Autodesk Inventor part; units mm, degrees
ref_plane "YZ Plane" through (0, 0, 0) normal (1, 0, 0) x (0, 1, 0)
ref_plane "XZ Plane" through (0, 0, 0) normal (0, 1, 0) x (-1, 0, 0)
ref_plane "XY Plane" through (0, 0, 0) normal (0, 0, 1) x (1, 0, 0)
sketch "Sketch1" plane through (0, 0, 0) normal (0, 1, 0) x (-1, 0, 0)
  line L0 (0, 0) -> (878.84, 0)
  line L1 (878.84, 0) -> (878.84, -66.04)
  line L2 (878.84, -66.04) -> (0, -66.04)
  line L3 (0, -66.04) -> (0, 0)
  line L4 (0, 0) -> (0, -20.32)
  line L5 (0, 0) -> (20.32, 0) construction
  line L6 (0, -20.32) -> (878.84, -20.32)
  line L7 (0, -10.16) -> (20.32, -10.16)
  line L8 (0, -10.16) -> (20.32, -10.16) construction
  circle A0 centre (20.32, -10.16) radius 2.54
  line L9 (20.32, -10.16) -> (172.72, -10.16)
  line L10 (20.32, -10.16) -> (172.72, -10.16) construction
  circle A1 centre (172.72, -10.16) radius 2.54
  line L11 (172.72, -10.16) -> (325.12, -10.16)
  circle A2 centre (325.12, -10.16) radius 2.54
  line L12 (325.12, -10.16) -> (477.52, -10.16)
  circle A3 centre (477.52, -10.16) radius 2.54
  line L13 (477.52, -10.16) -> (629.92, -10.16)
  circle A4 centre (629.92, -10.16) radius 2.54
  line L14 (629.92, -10.16) -> (782.32, -10.16)
  circle A5 centre (782.32, -10.16) radius 2.54
  line L15 (878.84, 0) -> (878.84, -10.16)
  line L16 (878.84, 0) -> (889, 0) construction
  line L17 (878.84, -10.16) -> (868.68, -10.16)
  circle A6 centre (868.68, -10.16) radius 2.54
  line L18 (0, 0) -> (0, -27.94)
  line L19 (0, 0) -> (27.94, 0) construction
  line L20 (0, -27.94) -> (27.94, -27.94)
  circle A7 centre (27.94, -27.94) radius 2.54
  line L21 (27.94, -27.94) -> (104.14, -27.94)
  line L22 (27.94, -27.94) -> (104.14, -27.94) construction
  circle A8 centre (104.14, -27.94) radius 2.54
  line L23 (104.14, -27.94) -> (129.54, -27.94)
  line L24 (142.24, -40.64) -> (142.24, -66.04)
  line L25 (142.24, -66.04) -> (116.84, -66.04)
  line L26 (116.84, -66.04) -> (116.84, -40.64)
  line L27 (116.84, -27.94) -> (116.84, -40.64)
  line L28 (116.84, -27.94) -> (129.54, -27.94) construction
  line L29 (116.84, -40.64) -> (129.54, -40.64)
  arc A9 (142.24, -40.64) -> (116.84, -40.64) centre (129.54, -40.64) ccw
  line L30 (142.24, -40.64) -> (154.94, -40.64) construction
  line L31 (142.24, -66.04) -> (154.94, -66.04)
  line L32 (142.24, -66.04) -> (154.94, -66.04) construction
  line L33 (154.94, -66.04) -> (154.94, -34.29)
  circle A10 centre (154.94, -34.29) radius 2.54
  line L34 (154.94, -34.29) -> (231.14, -34.29)
  line L35 (154.94, -34.29) -> (231.14, -34.29) construction
  circle A11 centre (231.14, -34.29) radius 2.54
  line L36 (154.94, -34.29) -> (104.14, -34.29)
  line L37 (154.94, -34.29) -> (205.74, -34.29) construction
  line L38 (269.24, -40.64) -> (269.24, -66.04)
  line L39 (243.84, -66.04) -> (243.84, -40.64)
  arc A12 (269.24, -40.64) -> (243.84, -40.64) centre (256.54, -40.64) ccw
  circle A13 centre (281.94, -34.29) radius 2.54
  line L40 (281.94, -34.29) -> (358.14, -34.29)
  circle A14 centre (358.14, -34.29) radius 2.54
  line L41 (281.94, -34.29) -> (231.14, -34.29)
  line L42 (396.24, -40.64) -> (396.24, -66.04)
  line L43 (370.84, -66.04) -> (370.84, -40.64)
  arc A15 (396.24, -40.64) -> (370.84, -40.64) centre (383.54, -40.64) ccw
  circle A16 centre (408.94, -34.29) radius 2.54
  line L44 (408.94, -34.29) -> (485.14, -34.29)
  circle A17 centre (485.14, -34.29) radius 2.54
  line L45 (408.94, -34.29) -> (358.14, -34.29)
  line L46 (523.24, -40.64) -> (523.24, -66.04)
  line L47 (497.84, -66.04) -> (497.84, -40.64)
  arc A18 (523.24, -40.64) -> (497.84, -40.64) centre (510.54, -40.64) ccw
  circle A19 centre (535.94, -34.29) radius 2.54
  line L48 (535.94, -34.29) -> (612.14, -34.29)
  circle A20 centre (612.14, -34.29) radius 2.54
  line L49 (535.94, -34.29) -> (485.14, -34.29)
  line L50 (650.24, -40.64) -> (650.24, -66.04)
  line L51 (624.84, -66.04) -> (624.84, -40.64)
  arc A21 (650.24, -40.64) -> (624.84, -40.64) centre (637.54, -40.64) ccw
  circle A22 centre (662.94, -34.29) radius 2.54
  line L52 (662.94, -34.29) -> (739.14, -34.29)
  circle A23 centre (739.14, -34.29) radius 2.54
  line L53 (662.94, -34.29) -> (612.14, -34.29)
  line L54 (777.24, -40.64) -> (777.24, -66.04)
  line L55 (751.84, -66.04) -> (751.84, -40.64)
  arc A24 (777.24, -40.64) -> (751.84, -40.64) centre (764.54, -40.64) ccw
  circle A25 centre (789.94, -34.29) radius 2.54
  line L56 (789.94, -34.29) -> (866.14, -34.29)
  circle A26 centre (866.14, -34.29) radius 2.54
  line L57 (789.94, -34.29) -> (739.14, -34.29)
  line L58 (0, -132.08) -> (878.84, -132.08)
  line L59 (878.84, -132.08) -> (878.84, -66.04)
  line L60 (0, -66.04) -> (0, -132.08)
  line L61 (0, -132.08) -> (0, -111.76)
  line L62 (0, -132.08) -> (20.32, -132.08) construction
  line L63 (0, -111.76) -> (878.84, -111.76)
  line L64 (0, -121.92) -> (20.32, -121.92)
  line L65 (0, -121.92) -> (20.32, -121.92) construction
  circle A27 centre (20.32, -121.92) radius 2.54
  line L66 (20.32, -121.92) -> (172.72, -121.92)
  line L67 (20.32, -121.92) -> (172.72, -121.92) construction
  circle A28 centre (172.72, -121.92) radius 2.54
  circle A29 centre (325.12, -121.92) radius 2.54
  line L68 (172.72, -121.92) -> (325.12, -121.92)
  circle A30 centre (477.52, -121.92) radius 2.54
  line L69 (325.12, -121.92) -> (477.52, -121.92)
  circle A31 centre (629.92, -121.92) radius 2.54
  line L70 (477.52, -121.92) -> (629.92, -121.92)
  circle A32 centre (782.32, -121.92) radius 2.54
  line L71 (629.92, -121.92) -> (782.32, -121.92)
  line L72 (878.84, -132.08) -> (878.84, -121.92)
  line L73 (878.84, -132.08) -> (889, -132.08) construction
  line L74 (878.84, -121.92) -> (868.68, -121.92)
  circle A33 centre (868.68, -121.92) radius 2.54
  line L75 (0, -132.08) -> (0, -104.14)
  line L76 (0, -132.08) -> (27.94, -132.08) construction
  line L77 (0, -104.14) -> (27.94, -104.14)
  circle A34 centre (27.94, -104.14) radius 2.54
  line L78 (27.94, -104.14) -> (104.14, -104.14)
  line L79 (27.94, -104.14) -> (104.14, -104.14) construction
  circle A35 centre (104.14, -104.14) radius 2.54
  line L80 (104.14, -104.14) -> (129.54, -104.14)
  line L81 (142.24, -91.44) -> (142.24, -66.04)
  line L82 (116.84, -66.04) -> (116.84, -91.44)
  line L83 (116.84, -104.14) -> (116.84, -91.44)
  line L84 (116.84, -104.14) -> (129.54, -104.14) construction
  line L85 (116.84, -91.44) -> (129.54, -91.44)
  arc A36 (116.84, -91.44) -> (142.24, -91.44) centre (129.54, -91.44) ccw
  line L86 (142.24, -91.44) -> (154.94, -91.44) construction
  line L87 (154.94, -66.04) -> (154.94, -97.79)
  circle A37 centre (154.94, -97.79) radius 2.54
  line L88 (154.94, -97.79) -> (231.14, -97.79)
  line L89 (154.94, -97.79) -> (231.14, -97.79) construction
  circle A38 centre (231.14, -97.79) radius 2.54
  line L90 (154.94, -97.79) -> (104.14, -97.79)
  line L91 (154.94, -97.79) -> (205.74, -97.79) construction
  line L92 (281.94, -97.79) -> (231.14, -97.79)
  line L93 (281.94, -97.79) -> (358.14, -97.79)
  line L94 (269.24, -91.44) -> (269.24, -66.04)
  line L95 (243.84, -66.04) -> (243.84, -91.44)
  arc A39 (243.84, -91.44) -> (269.24, -91.44) centre (256.54, -91.44) ccw
  circle A40 centre (281.94, -97.79) radius 2.54
  circle A41 centre (358.14, -97.79) radius 2.54
  line L96 (408.94, -97.79) -> (358.14, -97.79)
  line L97 (408.94, -97.79) -> (485.14, -97.79)
  line L98 (396.24, -91.44) -> (396.24, -66.04)
  line L99 (370.84, -66.04) -> (370.84, -91.44)
  arc A42 (370.84, -91.44) -> (396.24, -91.44) centre (383.54, -91.44) ccw
  circle A43 centre (408.94, -97.79) radius 2.54
  circle A44 centre (485.14, -97.79) radius 2.54
  line L100 (535.94, -97.79) -> (485.14, -97.79)
  line L101 (535.94, -97.79) -> (612.14, -97.79)
  line L102 (523.24, -91.44) -> (523.24, -66.04)
  line L103 (497.84, -66.04) -> (497.84, -91.44)
  arc A45 (497.84, -91.44) -> (523.24, -91.44) centre (510.54, -91.44) ccw
  circle A46 centre (535.94, -97.79) radius 2.54
  circle A47 centre (612.14, -97.79) radius 2.54
  line L104 (662.94, -97.79) -> (612.14, -97.79)
  line L105 (662.94, -97.79) -> (739.14, -97.79)
  line L106 (650.24, -91.44) -> (650.24, -66.04)
  line L107 (624.84, -66.04) -> (624.84, -91.44)
  arc A48 (624.84, -91.44) -> (650.24, -91.44) centre (637.54, -91.44) ccw
  circle A49 centre (662.94, -97.79) radius 2.54
  circle A50 centre (739.14, -97.79) radius 2.54
  line L108 (789.94, -97.79) -> (739.14, -97.79)
  line L109 (789.94, -97.79) -> (866.14, -97.79)
  line L110 (777.24, -91.44) -> (777.24, -66.04)
  line L111 (751.84, -66.04) -> (751.84, -91.44)
  arc A51 (751.84, -91.44) -> (777.24, -91.44) centre (764.54, -91.44) ccw
  circle A52 centre (789.94, -97.79) radius 2.54
  circle A53 centre (866.14, -97.79) radius 2.54
  dimension "d8" = 878.84
  dimension "d9" = 66.04
  dimension "d10" = 20.32
  dimension "d11" = 90
  dimension "d12" = 878.84
  dimension "d14" = 20.32
  dimension "d15" = 0
  dimension "d16" = 5.08
  dimension "d17" = 152.4
  dimension "d19" = 5.08
  dimension "d20" = 152.4
  dimension "d21" = 5.08
  dimension "d22" = 152.4
  dimension "d23" = 5.08
  dimension "d24" = 152.4
  dimension "d25" = 5.08
  dimension "d26" = 152.4
  dimension "d27" = 5.08
  dimension "d28" = 10.16
  dimension "d29" = 90
  dimension "d30" = 10.16
  dimension "d31" = 90
  dimension "d32" = 5.08
  dimension "d33" = 27.94
  dimension "d34" = 90
  dimension "d35" = 27.94
  dimension "d36" = 90
  dimension "d37" = 5.08
  dimension "d38" = 76.2
  dimension "d39" = 0
  dimension "d40" = 5.08
  dimension "d41" = 25.4
  dimension "d43" = 25.4
  dimension "d46" = 12.7
  dimension "d47" = 90
  dimension "d48" = 12.7
  dimension "d51" = 12.7
  dimension "d52" = 0
  dimension "d53" = 31.75
  dimension "d54" = 90
  dimension "d55" = 5.08
  dimension "d56" = 76.2
  dimension "d57" = 0
  dimension "d58" = 5.08
  dimension "d59" = 50.8
  dimension "d60" = 180
  dimension "d61" = 25.4
  dimension "d62" = 5.08
  dimension "d63" = 76.2
  dimension "d64" = 5.08
  dimension "d65" = 50.8
  dimension "d66" = 25.4
  dimension "d67" = 5.08
  dimension "d68" = 76.2
  dimension "d69" = 5.08
  dimension "d70" = 50.8
  dimension "d71" = 25.4
  dimension "d72" = 5.08
  dimension "d73" = 76.2
  dimension "d74" = 5.08
  dimension "d75" = 50.8
  dimension "d76" = 25.4
  dimension "d77" = 5.08
  dimension "d78" = 76.2
extrude "Extrusion1" add sketch "Sketch1" along normal blind 3.175 contours L0 L1 L6 L3 | L6 L1 L2 L54 A24 L57 A23 L52 A22 L53 A21 A20 L48 A19 L49 A18 A17 L44 A16 L45 A15 A14 L40 A13 L41 A12 A11 L34 A10 L36 A9 L23 A8 L21 A7 L20 L3 | L20 A7 L21 A8 L23 L27 L26 L2 L3 | L59 L63 L60 L77 A34 L78 A35 L80 A36 L90 A37 L88 A38 L92 A39 A40 L93 A41 L96 A42 A43 L97 A44 L100 A45 A46 L101 A47 L104 A48 A49 L105 A50 L108 A51 L110 L2 | L2 L82 L83 L80 A35 L78 A34 L77 L60 | L59 L58 L60 L63 | L111 A51 L108 A50 L105 A49 L104 A48 L106 L2 | L2 L50 A21 L53 A22 L52 A23 L57 A24 L55 | L24 A9 L36 A10 L33 L2 | L2 L87 A37 L90 A36 L81 | L27 L36 A9 | A36 L90 L83 | L33 A10 L34 A11 L41 A12 L39 L2 | L2 L95 A39 L92 A38 L88 A37 L87 | L27 L23 A9 L36 | L90 A36 L80 L83 | L107 A48 L104 A47 L101 A46 L100 A45 L102 L2 | L2 L46 A18 L49 A19 L48 A20 L53 A21 L51 | L38 A12 L41 A13 L40 A14 L45 A15 L43 L2 | L2 L99 A42 L96 A41 L93 A40 L92 A39 L94 | L103 A45 L100 A44 L97 A43 L96 A42 L98 L2 | L2 L42 A15 L45 A16 L44 A17 L49 A18 L47
properties part number "PCBMountingPlate"
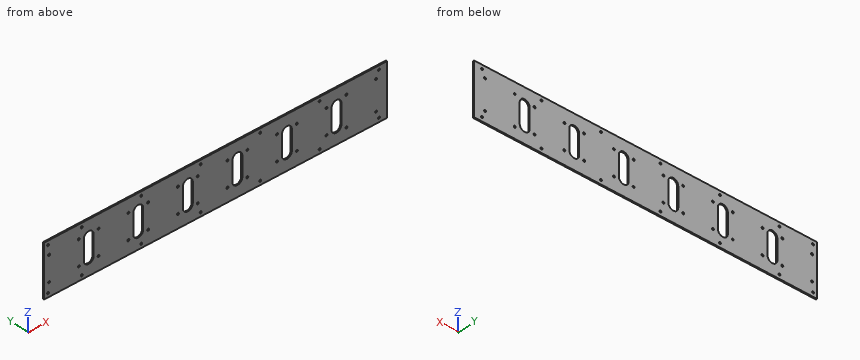
Check sheet for the modelled part. Datum: model origin and axes. Units: mm. Give positions to 0.01 mm unless a question says otherwise; leave off trailing zeros. Order: outer loops, then holes, each group sorted by start corner. A loop starts at its lowest first (then second) coordinate and runs counter-clockwise, first axis right, second up. Notation, with made-up numbers: (56.25, 33) -> (87.25, 33) arc R14 ccw to (87.25, 53) -> close; hole circle Ø9 at (-39.75, 55). An arc over 180 degrees is marked (long way). Return JSON: item names as keys, results as strings.
1. Material ranges on probe 1 along Z at (x, y) = (-478, 0.4); probe 2 along Z at (x, y) = (-231.14, 0.85); probe 3 along Z at (x, y) = (-772.5, 2.85), recorded low to high. Write a range as [from, to].
From the geometry:
{"probe 1": "[-132.08, -124.41], [-119.43, -12.65], [-7.67, 0]", "probe 2": "[-132.08, -100.33], [-95.25, -36.83], [-31.75, 0]", "probe 3": "[-132.08, -101.34], [-30.74, 0]"}
2. Cross-section at C-C, the plane y = 1.6. Count the separate pieces of the cut face and the enclosed holes in it, plus the area to 3 significant figures.
From the geometry:
{"separate pieces": "1", "enclosed holes": "48", "area": "104,000 mm^2"}
3. Cross-section at B-B, the plane x = -256.54. Record the cut outline in (y, z) (3 decimals).
From the geometry:
{"outline": "(0, -132.08) -> (3.175, -132.08) -> (3.175, -104.14) -> (0, -104.14) -> close; (0, -27.94) -> (3.175, -27.94) -> (3.175, 0) -> (0, 0) -> close"}
4. Cross-section at A-A, the plane z = -83. Record the cut outline in (x, y) (3 decimals), plus the area to 3 significant figures.
From the geometry:
{"outline": "(-878.84, 0) -> (-777.24, 0) -> (-777.24, 3.175) -> (-878.84, 3.175) -> close; (-751.84, 0) -> (-650.24, 0) -> (-650.24, 3.175) -> (-751.84, 3.175) -> close; (-624.84, 0) -> (-523.24, 0) -> (-523.24, 3.175) -> (-624.84, 3.175) -> close; (-497.84, 0) -> (-396.24, 0) -> (-396.24, 3.175) -> (-497.84, 3.175) -> close; (-370.84, 0) -> (-269.24, 0) -> (-269.24, 3.175) -> (-370.84, 3.175) -> close; (-243.84, 0) -> (-142.24, 0) -> (-142.24, 3.175) -> (-243.84, 3.175) -> close; (-116.84, 0) -> (0, 0) -> (0, 3.175) -> (-116.84, 3.175) -> close", "area": "2,310 mm^2"}
